```python
from build123d import *

# Parameters (mm, degrees)
F1_DEPTH = 1.5


# Not quite as in the source:
# - ends of sketch curves that miss each other by under 0.0002 mm in the source are joined


with BuildPart() as f1:
    # F0 (on Top) → F1 (new body)
    with BuildSketch(Plane.XY):
        Polygon((-154.7862010079, -56.3197720771), (-155.698514, -56.31515), (-156.1119683507, -57.0229680515), (-188.1119961072, -0.943063637), (-252.2166275849, -110.6877438524), (-187.6499915883, -111.0148592346), (-188.0469170019, -111.6943803821), (-187.578521744, -112.5152405744), (-252.1451579752, -112.188125191), (-189.1969680657, -222.5045451407), (-156.6379224358, -166.7385013741), (-156.261298, -167.398534), (-155.2892116972, -167.4034589083), (-187.8405636484, -223.1563251995), (-60.9469641109, -223.7992090591), (-92.9469916323, -167.7193050566), (-92.127277, -167.723458), (-91.6671171884, -166.9356819838), (-59.667332984, -223.0151595742), (4.3105823215, -113.4874126049), (-60.2555620411, -113.1602997135), (-59.778874, -112.344228), (-60.1688938721, -111.6607195518), (4.3977421328, -111.987834934), (-58.5385800691, -1.6922148149), (-90.9212471101, -57.156163237), (-91.0976251965, -57.4582577209), (-91.4381361233, -56.861513861), (-91.8289476292, -56.638734186), (-92.3545377772, -56.6360713738), (-59.8031858283, -0.8832050865), (-186.7862285296, -0.239868074), (-155.0159777331, -55.9170894017), align=None)
        Polygon((-124.7326106109, -112.0151510591), (-124.6877867318, -112.0153781513), (-124.7103900886, -112.0540924243), align=None, mode=Mode.SUBTRACT)
        Polygon((-123.0005820296, -112.023926074), (-122.955962742, -112.0241521297), (-122.9784629293, -112.0626896976), align=None, mode=Mode.SUBTRACT)
    extrude(amount=F1_DEPTH)


solid = f1.part
```
CAD build for the part. Positions are in the model's coordinates, mm. A direction names the side the tool comes from. Coordinates: 2 decimals unless noted, no trailing zeros. Order: outer loops, then holes, each group sorted by start corner. A loop starts at its lowest first (then second) coordinate and runs counter-clockwise, first axis right, second up.
(1) Drill centre lines: L1, parallel to Y at x = -69, z = 1.25; L2, parallel to X at y = -175, z = 0.7; L3, parallel to Y at x = -170.5, z = 1.15. Where is each one in solid material? Low to high.
Solution:
L1: y = -223.76 to -209.69, -206.66 to -19.61, -16.64 to -0.84
L2: x = -216.3 to -161.46, -159.72 to -88.79, -87.07 to -31.62
L3: y = -223.24 to -193.46, -190.48 to -31.81, -28.78 to -0.32
(2) Saw through at B-B, the plane x = -26. Write the cut outline in (y, z).
Solution:
outline: (-165.38, 0) - (-113.33, 0) - (-113.33, 1.5) - (-165.38, 1.5) - close; (-111.83, 0) - (-58.72, 0) - (-58.72, 1.5) - (-111.83, 1.5) - close
(3) Which spindle directions (+Z, -Z, +X, -X, +Y, -Y) get a long thin tool onto all of the face, cutting with end or side? Do faces 1 (the face through (-221.112, -166.574, 0.74)), 2 (the face through (-75.891, -194.583, 0.74)). Say none if no direction does.
Solution:
face 1: +Z, -Z, -X, -Y
face 2: +Z, -Z
(4) Mould opens along Y. For faces 3 (the face through (-219.716, -55.047, 0.74)), 4 (the face through (-28.126, -169.018, 0.74)), 5 (the face through (-126, -110, 0)), 6 (the face through (-173.145, -195.012, 0.74)) say: released by +Y, released by -Y, zero draft, split by the parting line, or undercut.
Solution:
face 3: released by +Y
face 4: released by -Y
face 5: zero draft
face 6: undercut
(5) Saw through at A-A, the plane y = -30. Write the cut outline in (x, z), and give its area (3 significant figures).
Solution:
outline: (-205.08, 0) - (-171.53, 0) - (-171.53, 1.5) - (-205.08, 1.5) - close; (-169.8, 0) - (-76.8, 0) - (-76.8, 1.5) - (-169.8, 1.5) - close; (-75.07, 0) - (-42.39, 0) - (-42.39, 1.5) - (-75.07, 1.5) - close
area: 239 mm2
(6) Saw through at D-D, the plane x = -86. Write the cut outline in (y, z).
Solution:
outline: (-223.67, 0) - (-179.89, 0) - (-179.89, 1.5) - (-223.67, 1.5) - close; (-176.87, 0) - (-48.73, 0) - (-48.73, 1.5) - (-176.87, 1.5) - close; (-45.75, 0) - (-0.75, 0) - (-0.75, 1.5) - (-45.75, 1.5) - close
